from build123d import *

# Parameters (mm, degrees)
BOSS_EXTRUDE1_DEPTH      = 40
SKETCH2_W                = 40
SKETCH2_H                = 29
BOSS_EXTRUDE2_DEPTH      = 23.5
SKETCH3_W                = 2.5
SKETCH3_H                = 8
CUT_EXTRUDE1_DEPTH       = 77.264342913
CUT_EXTRUDE2_REACH       = 76.863
SKETCH4_W                = 10
SKETCH4_H                = 29
CUT_EXTRUDE3_DEPTH       = 75.863208587
FILLET1_R                = 20
SKETCH6_R                = 2
CUT_EXTRUDE4_DEPTH       = 15.25
CUT_EXTRUDE5_REACH       = 78.264
SKETCH7_R                = 1.75
SKETCH8_R                = 3
CUT_EXTRUDE6_DEPTH       = 1
BOSS_EXTRUDE4_DEPTH      = 2
BOSS_EXTRUDE4_DEPTH_BACK = 2
CHAMFER1_SIZE            = 3
CHAMFER1_SIZE2           = 5
CHAMFER2_SIZE            = 5
CHAMFER2_SIZE2           = 3
CHAMFER3_SIZE            = 3
CHAMFER4_SIZE            = 3
CUT_EXTRUDE7_REACH       = 70.558
BOSS_EXTRUDE5_REACH      = 73.114
SKETCH12_W               = 10
SKETCH12_H               = 11.25
CUT_EXTRUDE8_DEPTH       = 2
FILLET2_R                = 1
SKETCH13_W               = 4.75
SKETCH13_H               = 32.080750089
CUT_EXTRUDE9_DEPTH       = 72.114344545
CUT_EXTRUDE10_REACH      = 76.305
SKETCH14_R               = 2


with BuildPart() as part:
    # Sketch1 → Boss-Extrude1 (new body)
    with BuildSketch(Plane(origin=(0, 0, 0), x_dir=(0, 0, -1), z_dir=(1, 0, 0))):
        Polygon((0, 0), (0, -56.5), (5, -56.5), (5, -5), (32, -5), (32, 0), align=None)
    extrude(amount=BOSS_EXTRUDE1_DEPTH)

    # Sketch2 → Boss-Extrude2 (add)
    with BuildSketch(Plane(origin=(0, 0, -5), x_dir=(-1, 0, 0), z_dir=(0, 0, -1))):
        with Locations((-20, -42)):
            Rectangle(SKETCH2_W, SKETCH2_H)
    extrude(amount=BOSS_EXTRUDE2_DEPTH)

    # Sketch3 → Cut-Extrude1 (cut, through all)
    with BuildSketch(Plane(origin=(40, 0, 0), x_dir=(0, 0, -1), z_dir=(1, 0, 0))):
        with Locations((18.5, -34.5)):
            Rectangle(SKETCH3_W, SKETCH3_H)
        with Locations((18.5, -48.5)):
            Rectangle(SKETCH3_W, SKETCH3_H)
    extrude(amount=-CUT_EXTRUDE1_DEPTH, mode=Mode.SUBTRACT)

    # Cut-Extrude2: up to this face of the body (flat: up to its plane)
    cut_extrude2_end = Plane(part.part.faces().sort_by_distance((20, -34.5, -17.25))[0])
    # Sketch4 → Cut-Extrude2 (cut, up to the picked face)
    with BuildSketch(Plane(origin=(0, 0, -28.5), x_dir=(-1, 0, 0), z_dir=(0, 0, -1)), mode=Mode.PRIVATE) as cut_extrude2_sk1:
        with Locations((-20, -42)):
            Rectangle(SKETCH4_W, SKETCH4_H)
    cut_extrude2_tool1 = split(extrude(cut_extrude2_sk1.sketch, amount=-CUT_EXTRUDE2_REACH, mode=Mode.PRIVATE), bisect_by=cut_extrude2_end, keep=Keep.BOTH, mode=Mode.PRIVATE)
    add(cut_extrude2_tool1.solids().sort_by(Axis((20, -42, -28.5), (0, 0, 1)))[0], mode=Mode.SUBTRACT)

    # Sketch5 → Cut-Extrude3 (cut, through all)
    with BuildSketch(Plane(origin=(0, 0, -28.5), x_dir=(-1, 0, 0), z_dir=(0, 0, -1))):
        Polygon((-29, -27.5), (-29, -56.5), (-40, -56.5), (-40, -13), align=None)
        Polygon((0, -56.5), (0, -13), (-11, -27.5), (-11, -56.5), align=None)
    extrude(amount=-CUT_EXTRUDE3_DEPTH, mode=Mode.SUBTRACT)

    # Fillet1
    fillet1_edges = [part.edges().sort_by_distance(p)[0] for p in [
        (40, -13, -2.5),
        (29, -27.5, -2.5),
        (11, -27.5, -2.5),
        (0, -13, -2.5),
    ]]
    fillet(fillet1_edges, radius=FILLET1_R)

    # Sketch6 → Cut-Extrude4 (cut)
    with BuildSketch(Plane(origin=(0, 0, -17.25), x_dir=(-1, 0, 0), z_dir=(0, 0, -1))):
        with Locations((-20, -42)):
            Circle(SKETCH6_R)
    extrude(amount=-CUT_EXTRUDE4_DEPTH, mode=Mode.SUBTRACT)

    # Sketch7 → Cut-Extrude5 (cut, up to next)
    with BuildSketch(Plane(origin=(0, 0, 0), x_dir=(1, 0, 0), z_dir=(0, 1, 0)), mode=Mode.PRIVATE) as cut_extrude5_sk1:
        with Locations(Location((30, 28.3, 0), (0, 0, 270))):
            Circle(SKETCH7_R)
    cut_extrude5_tool1 = extrude(cut_extrude5_sk1.sketch, amount=-CUT_EXTRUDE5_REACH, mode=Mode.PRIVATE) & part.part
    # Sketch7 → Cut-Extrude5 (cut, up to next)
    with BuildSketch(Plane(origin=(0, 0, 0), x_dir=(1, 0, 0), z_dir=(0, 1, 0)), mode=Mode.PRIVATE) as cut_extrude5_sk2:
        with Locations(Location((30, 8.3, 0), (0, 0, 270))):
            Circle(SKETCH7_R)
    cut_extrude5_tool2 = extrude(cut_extrude5_sk2.sketch, amount=-CUT_EXTRUDE5_REACH, mode=Mode.PRIVATE) & part.part
    # Sketch7 → Cut-Extrude5 (cut, up to next)
    with BuildSketch(Plane(origin=(0, 0, 0), x_dir=(1, 0, 0), z_dir=(0, 1, 0)), mode=Mode.PRIVATE) as cut_extrude5_sk3:
        with Locations(Location((10, 8.3, 0), (0, 0, 270))):
            Circle(SKETCH7_R)
    cut_extrude5_tool3 = extrude(cut_extrude5_sk3.sketch, amount=-CUT_EXTRUDE5_REACH, mode=Mode.PRIVATE) & part.part
    # Sketch7 → Cut-Extrude5 (cut, up to next)
    with BuildSketch(Plane(origin=(0, 0, 0), x_dir=(1, 0, 0), z_dir=(0, 1, 0)), mode=Mode.PRIVATE) as cut_extrude5_sk4:
        with Locations(Location((10, 28.3, 0), (0, 0, 270))):
            Circle(SKETCH7_R)
    cut_extrude5_tool4 = extrude(cut_extrude5_sk4.sketch, amount=-CUT_EXTRUDE5_REACH, mode=Mode.PRIVATE) & part.part
    add(cut_extrude5_tool1.solids().sort_by_distance((30, 0, -28.3))[0], mode=Mode.SUBTRACT)
    add(cut_extrude5_tool2.solids().sort_by_distance((30, 0, -8.3))[0], mode=Mode.SUBTRACT)
    add(cut_extrude5_tool3.solids().sort_by_distance((10, 0, -8.3))[0], mode=Mode.SUBTRACT)
    add(cut_extrude5_tool4.solids().sort_by_distance((10, 0, -28.3))[0], mode=Mode.SUBTRACT)

    # Sketch8 → Cut-Extrude6 (cut)
    with BuildSketch(Plane(origin=(0, 0, 0), x_dir=(1, 0, 0), z_dir=(0, 1, 0))):
        with Locations(Location((30, 28.3, 0), (0, 0, 270))):
            Circle(SKETCH8_R)
        with Locations(Location((30, 8.3, 0), (0, 0, 270))):
            Circle(SKETCH8_R)
        with Locations(Location((10, 8.3, 0), (0, 0, 270))):
            Circle(SKETCH8_R)
        with Locations(Location((10, 28.3, 0), (0, 0, 270))):
            Circle(SKETCH8_R)
    extrude(amount=-CUT_EXTRUDE6_DEPTH, mode=Mode.SUBTRACT)

    # Sketch9 → Boss-Extrude4 (add, two sides: drawn at the far end of the back side and taken through both)
    with BuildSketch(Plane.ZY.offset(-20).offset(-BOSS_EXTRUDE4_DEPTH_BACK)):
        Polygon((-32, 0), (0, 0), (0, -56.5), (3, -56.5), (3, 3), (-32, 3), align=None)
    extrude(amount=BOSS_EXTRUDE4_DEPTH + BOSS_EXTRUDE4_DEPTH_BACK)

    # Chamfer1
    chamfer1_edges = [part.edges().sort_by_distance(p)[0] for p in [
        (20, 3, -32),
    ]]
    chamfer1_side = [part.faces().sort_by_distance(p)[0] for p in [
        (20, -2.273584906, -32),
    ]]
    chamfer(chamfer1_edges, length=CHAMFER1_SIZE, length2=CHAMFER1_SIZE2, reference=chamfer1_side[0])

    # Chamfer2
    chamfer2_edges = [part.edges().sort_by_distance(p)[0] for p in [
        (20, -56.5, 3),
    ]]
    chamfer2_side = [part.faces().sort_by_distance(p)[0] for p in [
        (20, -26.75, 3),
    ]]
    chamfer(chamfer2_edges, length=CHAMFER2_SIZE, length2=CHAMFER2_SIZE2, reference=chamfer2_side[0])

    # Chamfer3
    chamfer3_edges = [part.edges().sort_by_distance(p)[0] for p in [
        (31, 0, 0),
        (9, 0, 0),
        (20, 3, 3),
    ]]
    chamfer(chamfer3_edges, length=CHAMFER3_SIZE)

    # Chamfer4
    chamfer4_edges = [part.edges().sort_by_distance(p)[0] for p in [
        (18, -29.75, 0),
        (18, -1.5, -1.5),
        (18, 0, -17.5),
        (22, -29.75, 0),
        (22, -1.5, -1.5),
        (22, 0, -17.5),
    ]]
    chamfer(chamfer4_edges, length=CHAMFER4_SIZE - 0.0001)  # a hair under: the kernel refuses the full size

    # Cut-Extrude7: up to this plane
    cut_extrude7_end = Plane(origin=(22, 0.621320344, 0.621320344), z_dir=(0.7071067811865434, 0.500000000000003, 0.500000000000003))
    # Sketch10 → Cut-Extrude7 (cut, up to the surface)
    with BuildSketch(Plane.ZY.offset(-18), mode=Mode.PRIVATE) as cut_extrude7_sk1:
        Polygon((-1.757359313, 3), (3, -1.757359313), (3, 0), (0, 3), align=None)
    cut_extrude7_tool1 = split(extrude(cut_extrude7_sk1.sketch, amount=-CUT_EXTRUDE7_REACH, mode=Mode.PRIVATE), bisect_by=cut_extrude7_end, keep=Keep.BOTH, mode=Mode.PRIVATE)
    add(cut_extrude7_tool1.solids().sort_by_distance((18, 1.027484, 1.027484))[0], mode=Mode.SUBTRACT)


with BuildPart() as cut_extrude7_kept_piece:
    # of the separate pieces the step leaves, the one the design keeps (cut_extrude7_pieces_kept)
    add(part.part.solids().sort_by_distance((18, -1.757400734, 2.9999))[0])

    # Boss-Extrude5: up to this face of the body (flat: up to its plane)
    boss_extrude5_end = Plane(cut_extrude7_kept_piece.part.faces().sort_by_distance((29, -42.52414206, -14.549200751))[0])
    # Sketch11 → Boss-Extrude5 (add, up to the picked face)
    with BuildSketch(Plane.ZY.offset(-11), mode=Mode.PRIVATE) as boss_extrude5_sk1:
        Polygon((-28.5, -27.5), (-9.859490986, -24.723753977), (-5, -16.5), (-5, -27.5), align=None)
    boss_extrude5_tool1 = split(extrude(boss_extrude5_sk1.sketch, amount=-BOSS_EXTRUDE5_REACH, mode=Mode.PRIVATE), bisect_by=boss_extrude5_end, keep=Keep.BOTH, mode=Mode.PRIVATE)
    add(boss_extrude5_tool1.solids().sort_by(Axis((11, -24.923314, -10.92545), (1, 0, 0)))[0])

    # Sketch12 → Cut-Extrude8 (cut)
    with BuildSketch(Plane.XZ.offset(27.5)):
        with Locations((20, -22.875)):
            Rectangle(SKETCH12_W, SKETCH12_H)
    extrude(amount=-CUT_EXTRUDE8_DEPTH, mode=Mode.SUBTRACT)

    # Fillet2
    fillet2_edges = [cut_extrude7_kept_piece.edges().sort_by_distance(p)[0] for p in [
        (29, -30.5, -18.5),
        (11, -34.5, -17.25),
        (11, -48.5, -17.25),
        (29, -38.5, -18.5),
        (29, -34.5, -19.75),
        (29, -34.5, -17.25),
        (29, -52.5, -18.5),
        (29, -48.5, -19.75),
        (29, -44.5, -18.5),
        (29, -48.5, -17.25),
        (11, -30.5, -18.5),
        (11, -34.5, -19.75),
        (11, -38.5, -18.5),
        (11, -44.5, -18.5),
        (11, -48.5, -19.75),
        (11, -52.5, -18.5),
        (25, -30.5, -18.5),
        (15, -30.5, -18.5),
        (15, -52.5, -18.5),
        (15, -48.5, -19.75),
        (15, -44.5, -18.5),
        (15, -38.5, -18.5),
        (15, -34.5, -19.75),
        (25, -48.5, -19.75),
        (25, -52.5, -18.5),
        (25, -34.5, -19.75),
        (25, -38.5, -18.5),
        (25, -44.5, -18.5),
    ]]
    fillet(fillet2_edges, radius=FILLET2_R)

    # Sketch13 → Cut-Extrude9 (cut, through all)
    with BuildSketch(Plane(origin=(29, 0, 0), x_dir=(0, 0, -1), z_dir=(1, 0, 0))):
        with Locations((26.125, -40.459624956)):
            Rectangle(SKETCH13_W, SKETCH13_H)
    extrude(amount=-CUT_EXTRUDE9_DEPTH, mode=Mode.SUBTRACT)

    # Sketch14 → Cut-Extrude10 (cut, up to next)
    with BuildSketch(Plane(origin=(0, 0, -5), x_dir=(-1, 0, 0), z_dir=(0, 0, -1)), mode=Mode.PRIVATE) as cut_extrude10_sk1:
        with Locations(Location((-32.5, -10.75, 0), (0, 0, 90))):
            Circle(SKETCH14_R)
    cut_extrude10_tool1 = extrude(cut_extrude10_sk1.sketch, amount=-CUT_EXTRUDE10_REACH, mode=Mode.PRIVATE) & cut_extrude7_kept_piece.part
    # Sketch14 → Cut-Extrude10 (cut, up to next)
    with BuildSketch(Plane(origin=(0, 0, -5), x_dir=(-1, 0, 0), z_dir=(0, 0, -1)), mode=Mode.PRIVATE) as cut_extrude10_sk2:
        with Locations(Location((-7.5, -10.75, 0), (0, 0, 90))):
            Circle(SKETCH14_R)
    cut_extrude10_tool2 = extrude(cut_extrude10_sk2.sketch, amount=-CUT_EXTRUDE10_REACH, mode=Mode.PRIVATE) & cut_extrude7_kept_piece.part
    add(cut_extrude10_tool1.solids().sort_by_distance((32.5, -10.75, -5))[0], mode=Mode.SUBTRACT)
    add(cut_extrude10_tool2.solids().sort_by_distance((7.5, -10.75, -5))[0], mode=Mode.SUBTRACT)


solid = cut_extrude7_kept_piece.part
CAD build for the part. Positions are in the model's coordinates, mm. A direction names the side the tool comes from. Give positions to 0.01 mm unless a question says otherwise; leave off trailing zeros. Write each loop counter-clockwise with the first axis right and the second up, starting at its lowest first coordinate (ties: lowest second). Pieces come first, ordered by that corner, then holes. Notation, with made-up numbers: M 11.25,-8.75 L 54.25,-8.75 A17 cw 54.25,15.25 Z; hole C 49.5,53.25 d4. An arc over 180 degrees is marked long. Put each result on its own line as item: value. Start each with the question number.
(1) Band-saw the part on B-B, the plane x = 20. Write the cut outline in (y, z), and give its area (3 significant figures).
(2) Probe L1, parallel to X at y = -0.55, z = -8.3; L2, parallel to Z at x = 13.5, y = -32; L3, parallel to Y at x = 3.5, z = -27.5. List the from-to ranges inside material, lowest first.
(3) Band-saw the part on A-A, the plane z = -8.3. Give the number of separate pieces and of enclosed holes in the cut face, and give its area (3 significant figures).
(4) Which spindle directions (+Z, -Z, +X, -X, +Y, -Y) get a long thin tool onto all of the face, cutting with end or side? Do faces 1 (the face through (32, 0, -18)), 2 (the face through (27, -42, -23.75)), 3 (the face through (27, -30.5, -18)), 4 (the face through (11, -41, -12)). Say none if no direction does.
(5) Flat gauge pins, fed straight in: pin 1 Ø5 at (x, z) = (22.5, -28.5) entering from -Y; pin 2 Ø6.5 at (x, z) = (9, -27.5) entering from +Y; pin 3 Ø2 at (x, y) = (28, -40.5) entering from -Z; pin 4 Ø23.5 at (x, y) = (15.5, -13.5) entering from -Z. Where does each tip first touch, or does it go through?
(6) Band-saw the part on D-D, the plane z = -28.3. Write the cut outline in (x, y), and give its area (3 significant figures).
(7) Mould opens along Y. For faces 5 (the face through (34.52, -20.224, -2.535)), 6 (the face through (20, -13, -5)), 7 (the face through (28, -1, -28)) say: +Y half, -Y half, draft (parallel to the pull), parting line (faces both ways), or undercut.
Response values:
1. outline: M -56.5,-17.25 L -44,-17.25 L -44,-2 L -40,-2 L -40,-17.25 L -25.82,-17.25 L -24.72,-9.86 L -16.5,-5 L -5,-5 L -5,-32 L 0,-32 L 3,-27 L 3,-1.76 L -1.76,3 L -51.5,3 L -56.5,0 Z
1. area: 1,010 mm2
2. L1: x = 0 to 7, 13 to 27, 33 to 40
2. L2: z = -23.75 to -19.75, -17.25 to 0
2. L3: y = -5 to 0
3. separate pieces: 4
3. enclosed holes: 1
3. area: 788 mm2
4. face 1: +Z, -Z, +X, +Y
4. face 2: -Z, +X, -X, -Y
4. face 3: +X, -X
4. face 4: -Z, -X, -Y
5. pin 1: stops at y = -5
5. pin 2: stops at y = 0
5. pin 3: stops at z = -23.75
5. pin 4: stops at z = -32
6. outline: M 0,-5 L 8.25,-5 L 8.25,-1 L 7,-1 L 7,0 L 0,0 Z; M 11.75,-5 L 28.25,-5 L 28.25,-1 L 27,-1 L 27,0 L 25,0 L 22.78,2.22 L 17.22,2.22 L 15,0 L 13,0 L 13,-1 L 11.75,-1 Z; M 31.75,-5 L 40,-5 L 40,0 L 33,0 L 33,-1 L 31.75,-1 Z
6. area: 177 mm2
7. face 5: -Y half
7. face 6: undercut
7. face 7: +Y half
